For this review, take the finished solid that the model builds, in its own axes (mm). A direction names the side the tool comes from. Round coordinates to 2 decimals unless told otherwise and drop trailing zeros.
1) Mouldability with a two-part tool opening along Z and no side actions: class faces 3 (the cylindrical face through (-5.82, 3.34, 10.6)), 4 (the cylindrical face through (6.06, -11.21, -5.83)), 5 (the flat face through (0, 0, 13)) as pulls with the +Z half, pulls with the -Z half, needs draft (parallel to the pull), parting line crosses it, or undercut.
2) Tool access review of faces 1 (the flat face through (-2.413, -7.3, 2.3)), 2 (the cylindrical face through (-4.701, 15.497, 3.441)): name each direction out of +Z, -Z, +X, -X, +Y, -Y from which nothing blocks a thin tool from reaching the whole face with its end or side.
3) Wall thickness on L1, parallel to Y at x = -2.25, z = 0 (3 decimals); L2, parallel to Y at x = 3.5, z = 0; L3, parallel to X at y = -11.5, z = -6 (3 decimals): over which ranges is each line inside the solid? List them lowest first.
4) Insertion check: pin 1 (8 mm diameter, centred on x = 9, y = 8.5, fed in from -Z); pin 2 (5 mm diameter, centred on x = 10, z = 2.5, fed in from -Y); pin 3 (6 mm diameter, centred on y = -6, z = 2, fed in from -X); pin 4 (8 mm diameter, centred on y = 0, z = 0, fed in from -X). Each pin has a flat end and moves straight along its axis. Give the tip position at first contact, or say it passes through.
```python
from build123d import *

# Parameters (mm, degrees)
SKETCH1_R           = 12.6365
BOSS_EXTRUDE1_DEPTH = 12.7
SKETCH2_R           = 15.875
BOSS_EXTRUDE2_DEPTH = 9.525
SKETCH3_R           = 11.1125
CUT_EXTRUDE1_DEPTH  = 7.112
SKETCH4_R           = 7.27458794
CUT_EXTRUDE2_DEPTH  = 0.2
SKETCH5_R           = 5.08
CUT_EXTRUDE3_DEPTH  = 27.952343479
CHAMFER1_SIZE       = 0.4


with BuildPart() as part:
    # Sketch1 → Boss-Extrude1 (new body)
    with BuildSketch(Plane(origin=(0, 0, 0), x_dir=(0, 0, -1), z_dir=(1, 0, 0))):
        Circle(SKETCH1_R)
    extrude(amount=BOSS_EXTRUDE1_DEPTH)

    # Sketch2 → Boss-Extrude2 (add)
    with BuildSketch(Plane.ZY):
        with Locations(Location((0, 0, 0), (0, 0, 180))):
            Circle(SKETCH2_R)
    extrude(amount=BOSS_EXTRUDE2_DEPTH)

    # Sketch3 → Cut-Extrude1 (cut)
    with BuildSketch(Plane.ZY.offset(9.525)):
        Circle(SKETCH3_R)
    extrude(amount=-CUT_EXTRUDE1_DEPTH, mode=Mode.SUBTRACT)

    # Sketch4 → Cut-Extrude2 (cut)
    with BuildSketch(Plane.ZY.offset(2.413)):
        Circle(SKETCH4_R)
    extrude(amount=-CUT_EXTRUDE2_DEPTH, mode=Mode.SUBTRACT)

    # Sketch5 → Cut-Extrude3 (cut, through all)
    with BuildSketch(Plane.ZY.offset(2.213)):
        Circle(SKETCH5_R)
    extrude(amount=-CUT_EXTRUDE3_DEPTH, mode=Mode.SUBTRACT)

    # Chamfer1
    chamfer1_edges = [part.edges().sort_by_distance(p)[0] for p in [
        (-9.525, 0, -11.1125),
        (12.7, 0, -5.08),
        (12.7, 0, 12.6365),
        (0, 0, 15.875),
        (-9.525, 0, 15.875),
    ]]
    chamfer(chamfer1_edges, length=CHAMFER1_SIZE)


solid = part.part
```
Response:
1. face 3: undercut
1. face 4: parting line crosses it
1. face 5: needs draft
2. face 1: -X
2. face 2: +X, -X
3. L1: y = -15.875 to -7.275, 7.275 to 15.875
3. L2: y = -12.64 to -5.08, 5.08 to 12.64
3. L3: x = -9.525 to 0
4. pin 1: stops at z = -11.81
4. pin 2: stops at y = -12.64
4. pin 3: stops at x = -2.41
4. pin 4: passes through
